from build123d import *

# Parameters (mm, degrees)
ESQUISSE1_W                  = 300
ESQUISSE1_H                  = 100
BOSS_EXTRU_1_DEPTH           = 1.5875
ESQUISSE2_W                  = 19.05
ESQUISSE2_H                  = 61.9
BOSS_EXTRU_2_DEPTH           = 1.5875
ESQUISSE3_W                  = 1.5875
ESQUISSE3_H                  = 61.9
BOSS_EXTRU_3_DEPTH           = 17.4625
ENL_V_MAT_EXTRU_1_REACH      = 5.175
ESQUISSE4_R                  = 1.5875
ENL_V_MAT_EXTRU_2_REACH      = 22.637
ESQUISSE5_R                  = 1.5875
ENL_V_MAT_EXTRU_3_REACH      = 22.637
ESQUISSE6_R                  = 1.5875
ESQUISSE7_R                  = 1.5875
ENL_V_MAT_EXTRU_4_DEPTH      = 297.825
ENL_V_MAT_EXTRU_4_DEPTH_BACK = 4.175


with BuildPart() as part:
    # Esquisse1 → Boss.-Extru.1 (new body)
    with BuildSketch(Plane.XY):
        with Locations((29.89832913, 31.147540984)):
            Rectangle(ESQUISSE1_W, ESQUISSE1_H)
    extrude(amount=BOSS_EXTRU_1_DEPTH)

    # Esquisse2 → Boss.-Extru.2 (add)
    with BuildSketch(Plane(origin=(0, 0, 0), x_dir=(-1, 0, 0), z_dir=(0, 0, -1))):
        with Locations((108.98917087, 31.147540984)):
            Rectangle(ESQUISSE2_W, ESQUISSE2_H)
        with Locations((-168.78582913, 31.147540984)):
            Rectangle(ESQUISSE2_W, ESQUISSE2_H)
    extrude(amount=BOSS_EXTRU_2_DEPTH)

    # Esquisse3 → Boss.-Extru.3 (add)
    with BuildSketch(Plane(origin=(0, 0, -1.5875), x_dir=(-1, 0, 0), z_dir=(0, 0, -1))):
        with Locations((-177.51707913, 31.147540984)):
            Rectangle(ESQUISSE3_W, ESQUISSE3_H)
        with Locations((117.72042087, 31.147540984)):
            Rectangle(ESQUISSE3_W, ESQUISSE3_H)
    extrude(amount=BOSS_EXTRU_3_DEPTH)

    # Esquisse4 → Enlèv. mat.-Extru.1 (cut, up to next)
    with BuildSketch(Plane(origin=(0, 0, -1.5875), x_dir=(-1, 0, 0), z_dir=(0, 0, -1)), mode=Mode.PRIVATE) as enl_v_mat_extru_1_sk1:
        with Locations((-167.99207913, 52.572540984)):
            Circle(ESQUISSE4_R)
    enl_v_mat_extru_1_tool1 = extrude(enl_v_mat_extru_1_sk1.sketch, amount=-ENL_V_MAT_EXTRU_1_REACH, mode=Mode.PRIVATE) & part.part
    add(enl_v_mat_extru_1_tool1.solids().sort_by_distance((167.992079, 52.572541, -1.5875))[0], mode=Mode.SUBTRACT)
    # Esquisse4 → Enlèv. mat.-Extru.1 (cut, up to next)
    with BuildSketch(Plane(origin=(0, 0, -1.5875), x_dir=(-1, 0, 0), z_dir=(0, 0, -1)), mode=Mode.PRIVATE) as enl_v_mat_extru_1_sk2:
        with Locations((-167.99207913, 9.722540984)):
            Circle(ESQUISSE4_R)
    enl_v_mat_extru_1_tool2 = extrude(enl_v_mat_extru_1_sk2.sketch, amount=-ENL_V_MAT_EXTRU_1_REACH, mode=Mode.PRIVATE) & part.part
    add(enl_v_mat_extru_1_tool2.solids().sort_by_distance((167.992079, 9.722541, -1.5875))[0], mode=Mode.SUBTRACT)
    # Esquisse4 → Enlèv. mat.-Extru.1 (cut, up to next)
    with BuildSketch(Plane(origin=(0, 0, -1.5875), x_dir=(-1, 0, 0), z_dir=(0, 0, -1)), mode=Mode.PRIVATE) as enl_v_mat_extru_1_sk3:
        with Locations((108.19542087, 52.572540984)):
            Circle(ESQUISSE4_R)
    enl_v_mat_extru_1_tool3 = extrude(enl_v_mat_extru_1_sk3.sketch, amount=-ENL_V_MAT_EXTRU_1_REACH, mode=Mode.PRIVATE) & part.part
    add(enl_v_mat_extru_1_tool3.solids().sort_by_distance((-108.195421, 52.572541, -1.5875))[0], mode=Mode.SUBTRACT)
    # Esquisse4 → Enlèv. mat.-Extru.1 (cut, up to next)
    with BuildSketch(Plane(origin=(0, 0, -1.5875), x_dir=(-1, 0, 0), z_dir=(0, 0, -1)), mode=Mode.PRIVATE) as enl_v_mat_extru_1_sk4:
        with Locations((108.19542087, 9.722540984)):
            Circle(ESQUISSE4_R)
    enl_v_mat_extru_1_tool4 = extrude(enl_v_mat_extru_1_sk4.sketch, amount=-ENL_V_MAT_EXTRU_1_REACH, mode=Mode.PRIVATE) & part.part
    add(enl_v_mat_extru_1_tool4.solids().sort_by_distance((-108.195421, 9.722541, -1.5875))[0], mode=Mode.SUBTRACT)

    # Esquisse5 → Enlèv. mat.-Extru.2 (cut, up to next)
    with BuildSketch(Plane.XY.offset(1.5875), mode=Mode.PRIVATE) as enl_v_mat_extru_2_sk1:
        with Locations((-108.19542087, -8.533709016)):
            Circle(ESQUISSE5_R)
    enl_v_mat_extru_2_tool1 = extrude(enl_v_mat_extru_2_sk1.sketch, amount=-ENL_V_MAT_EXTRU_2_REACH, mode=Mode.PRIVATE) & part.part
    add(enl_v_mat_extru_2_tool1.solids().sort_by_distance((-108.195421, -8.533709, 1.5875))[0], mode=Mode.SUBTRACT)
    # Esquisse5 → Enlèv. mat.-Extru.2 (cut, up to next)
    with BuildSketch(Plane.XY.offset(1.5875), mode=Mode.PRIVATE) as enl_v_mat_extru_2_sk2:
        with Locations((-89.93917087, -8.533709016)):
            Circle(ESQUISSE5_R)
    enl_v_mat_extru_2_tool2 = extrude(enl_v_mat_extru_2_sk2.sketch, amount=-ENL_V_MAT_EXTRU_2_REACH, mode=Mode.PRIVATE) & part.part
    add(enl_v_mat_extru_2_tool2.solids().sort_by_distance((-89.939171, -8.533709, 1.5875))[0], mode=Mode.SUBTRACT)
    # Esquisse5 → Enlèv. mat.-Extru.2 (cut, up to next)
    with BuildSketch(Plane.XY.offset(1.5875), mode=Mode.PRIVATE) as enl_v_mat_extru_2_sk3:
        with Locations((-30.02042087, -8.533709016)):
            Circle(ESQUISSE5_R)
    enl_v_mat_extru_2_tool3 = extrude(enl_v_mat_extru_2_sk3.sketch, amount=-ENL_V_MAT_EXTRU_2_REACH, mode=Mode.PRIVATE) & part.part
    add(enl_v_mat_extru_2_tool3.solids().sort_by_distance((-30.020421, -8.533709, 1.5875))[0], mode=Mode.SUBTRACT)
    # Esquisse5 → Enlèv. mat.-Extru.2 (cut, up to next)
    with BuildSketch(Plane.XY.offset(1.5875), mode=Mode.PRIVATE) as enl_v_mat_extru_2_sk4:
        with Locations((29.89832913, -8.533709016)):
            Circle(ESQUISSE5_R)
    enl_v_mat_extru_2_tool4 = extrude(enl_v_mat_extru_2_sk4.sketch, amount=-ENL_V_MAT_EXTRU_2_REACH, mode=Mode.PRIVATE) & part.part
    add(enl_v_mat_extru_2_tool4.solids().sort_by_distance((29.898329, -8.533709, 1.5875))[0], mode=Mode.SUBTRACT)
    # Esquisse5 → Enlèv. mat.-Extru.2 (cut, up to next)
    with BuildSketch(Plane.XY.offset(1.5875), mode=Mode.PRIVATE) as enl_v_mat_extru_2_sk5:
        with Locations((89.81707913, -8.533709016)):
            Circle(ESQUISSE5_R)
    enl_v_mat_extru_2_tool5 = extrude(enl_v_mat_extru_2_sk5.sketch, amount=-ENL_V_MAT_EXTRU_2_REACH, mode=Mode.PRIVATE) & part.part
    add(enl_v_mat_extru_2_tool5.solids().sort_by_distance((89.817079, -8.533709, 1.5875))[0], mode=Mode.SUBTRACT)
    # Esquisse5 → Enlèv. mat.-Extru.2 (cut, up to next)
    with BuildSketch(Plane.XY.offset(1.5875), mode=Mode.PRIVATE) as enl_v_mat_extru_2_sk6:
        with Locations((149.73582913, -8.533709016)):
            Circle(ESQUISSE5_R)
    enl_v_mat_extru_2_tool6 = extrude(enl_v_mat_extru_2_sk6.sketch, amount=-ENL_V_MAT_EXTRU_2_REACH, mode=Mode.PRIVATE) & part.part
    add(enl_v_mat_extru_2_tool6.solids().sort_by_distance((149.735829, -8.533709, 1.5875))[0], mode=Mode.SUBTRACT)
    # Esquisse5 → Enlèv. mat.-Extru.2 (cut, up to next)
    with BuildSketch(Plane.XY.offset(1.5875), mode=Mode.PRIVATE) as enl_v_mat_extru_2_sk7:
        with Locations((167.99207913, -8.533709016)):
            Circle(ESQUISSE5_R)
    enl_v_mat_extru_2_tool7 = extrude(enl_v_mat_extru_2_sk7.sketch, amount=-ENL_V_MAT_EXTRU_2_REACH, mode=Mode.PRIVATE) & part.part
    add(enl_v_mat_extru_2_tool7.solids().sort_by_distance((167.992079, -8.533709, 1.5875))[0], mode=Mode.SUBTRACT)
    # Esquisse5 → Enlèv. mat.-Extru.2 (cut, up to next)
    with BuildSketch(Plane.XY.offset(1.5875), mode=Mode.PRIVATE) as enl_v_mat_extru_2_sk8:
        with Locations((167.99207913, 70.828790984)):
            Circle(ESQUISSE5_R)
    enl_v_mat_extru_2_tool8 = extrude(enl_v_mat_extru_2_sk8.sketch, amount=-ENL_V_MAT_EXTRU_2_REACH, mode=Mode.PRIVATE) & part.part
    add(enl_v_mat_extru_2_tool8.solids().sort_by_distance((167.992079, 70.828791, 1.5875))[0], mode=Mode.SUBTRACT)
    # Esquisse5 → Enlèv. mat.-Extru.2 (cut, up to next)
    with BuildSketch(Plane.XY.offset(1.5875), mode=Mode.PRIVATE) as enl_v_mat_extru_2_sk9:
        with Locations((149.73582913, 70.828790984)):
            Circle(ESQUISSE5_R)
    enl_v_mat_extru_2_tool9 = extrude(enl_v_mat_extru_2_sk9.sketch, amount=-ENL_V_MAT_EXTRU_2_REACH, mode=Mode.PRIVATE) & part.part
    add(enl_v_mat_extru_2_tool9.solids().sort_by_distance((149.735829, 70.828791, 1.5875))[0], mode=Mode.SUBTRACT)
    # Esquisse5 → Enlèv. mat.-Extru.2 (cut, up to next)
    with BuildSketch(Plane.XY.offset(1.5875), mode=Mode.PRIVATE) as enl_v_mat_extru_2_sk10:
        with Locations((89.81707913, 70.828790984)):
            Circle(ESQUISSE5_R)
    enl_v_mat_extru_2_tool10 = extrude(enl_v_mat_extru_2_sk10.sketch, amount=-ENL_V_MAT_EXTRU_2_REACH, mode=Mode.PRIVATE) & part.part
    add(enl_v_mat_extru_2_tool10.solids().sort_by_distance((89.817079, 70.828791, 1.5875))[0], mode=Mode.SUBTRACT)
    # Esquisse5 → Enlèv. mat.-Extru.2 (cut, up to next)
    with BuildSketch(Plane.XY.offset(1.5875), mode=Mode.PRIVATE) as enl_v_mat_extru_2_sk11:
        with Locations((29.89832913, 70.828790984)):
            Circle(ESQUISSE5_R)
    enl_v_mat_extru_2_tool11 = extrude(enl_v_mat_extru_2_sk11.sketch, amount=-ENL_V_MAT_EXTRU_2_REACH, mode=Mode.PRIVATE) & part.part
    add(enl_v_mat_extru_2_tool11.solids().sort_by_distance((29.898329, 70.828791, 1.5875))[0], mode=Mode.SUBTRACT)
    # Esquisse5 → Enlèv. mat.-Extru.2 (cut, up to next)
    with BuildSketch(Plane.XY.offset(1.5875), mode=Mode.PRIVATE) as enl_v_mat_extru_2_sk12:
        with Locations((-30.02042087, 70.828790984)):
            Circle(ESQUISSE5_R)
    enl_v_mat_extru_2_tool12 = extrude(enl_v_mat_extru_2_sk12.sketch, amount=-ENL_V_MAT_EXTRU_2_REACH, mode=Mode.PRIVATE) & part.part
    add(enl_v_mat_extru_2_tool12.solids().sort_by_distance((-30.020421, 70.828791, 1.5875))[0], mode=Mode.SUBTRACT)
    # Esquisse5 → Enlèv. mat.-Extru.2 (cut, up to next)
    with BuildSketch(Plane.XY.offset(1.5875), mode=Mode.PRIVATE) as enl_v_mat_extru_2_sk13:
        with Locations((-89.93917087, 70.828790984)):
            Circle(ESQUISSE5_R)
    enl_v_mat_extru_2_tool13 = extrude(enl_v_mat_extru_2_sk13.sketch, amount=-ENL_V_MAT_EXTRU_2_REACH, mode=Mode.PRIVATE) & part.part
    add(enl_v_mat_extru_2_tool13.solids().sort_by_distance((-89.939171, 70.828791, 1.5875))[0], mode=Mode.SUBTRACT)
    # Esquisse5 → Enlèv. mat.-Extru.2 (cut, up to next)
    with BuildSketch(Plane.XY.offset(1.5875), mode=Mode.PRIVATE) as enl_v_mat_extru_2_sk14:
        with Locations((-108.19542087, 70.828790984)):
            Circle(ESQUISSE5_R)
    enl_v_mat_extru_2_tool14 = extrude(enl_v_mat_extru_2_sk14.sketch, amount=-ENL_V_MAT_EXTRU_2_REACH, mode=Mode.PRIVATE) & part.part
    add(enl_v_mat_extru_2_tool14.solids().sort_by_distance((-108.195421, 70.828791, 1.5875))[0], mode=Mode.SUBTRACT)

    # Esquisse6 → Enlèv. mat.-Extru.3 (cut, up to next)
    with BuildSketch(Plane.XY.offset(1.5875), mode=Mode.PRIVATE) as enl_v_mat_extru_3_sk1:
        with Locations((19.89832913, 31.147540984)):
            Circle(ESQUISSE6_R)
    enl_v_mat_extru_3_tool1 = extrude(enl_v_mat_extru_3_sk1.sketch, amount=-ENL_V_MAT_EXTRU_3_REACH, mode=Mode.PRIVATE) & part.part
    add(enl_v_mat_extru_3_tool1.solids().sort_by_distance((19.898329, 31.147541, 1.5875))[0], mode=Mode.SUBTRACT)

    # Esquisse7 → Enlèv. mat.-Extru.4 (cut, two sides)
    with BuildSketch(Plane.ZY.offset(-176.72332913)) as enl_v_mat_extru_4_sk:
        with Locations((-10.31875, 52.572540984)):
            Circle(ESQUISSE7_R)
        with Locations((-10.31875, 9.722540984)):
            Circle(ESQUISSE7_R)
    extrude(amount=ENL_V_MAT_EXTRU_4_DEPTH, mode=Mode.SUBTRACT)
    extrude(enl_v_mat_extru_4_sk.sketch, amount=-ENL_V_MAT_EXTRU_4_DEPTH_BACK, mode=Mode.SUBTRACT)


solid = part.part
For this review, take the finished solid that the model builds, in its own axes (mm). A direction names the side the tool comes from. Round coordinates to 2 decimals unless told otherwise and drop trailing zeros. Loops run counter-clockwise (first coordinate to the right, second up) from the corner with the lowest first, then second, coordinate; pieces in that order, holes last. Notation, with made-up numbers: (78.5, 21) - (85.5, 21) arc R5 ccw to (85.5, 28) - close; hole circle Ø11 at (-28, 76.25). An arc over 180 degrees is marked (long way). One line per item, written item: value. Start each with the question number.
Item 1: Take a section at B-B (z = -15.75). Give the boundary of the cut face in (x, y).
Item 2: The part is to be moulded in two halves that separate along X. For faces 5 (the flat face through (-113, 62.098, -1)), 6 (the flat face through (28, 32, 0)), 7 (the flat face through (178.311, 31, -9)), 8 (the flat face through (-118.514, 31, -9)), say which applies: +X half, -X half, draft (parallel to the pull), parting line (faces both ways), or undercut.
Item 3: For faces 1 (the flat face through (-116.927, 31, -10)), 2 (the flat face through (-113, 0.198, -1)), 3 (the flat face through (177, 62.098, -5)), 4 (the flat face through (28, 32, 1.588)), list the 3-axis set-ups (+Z, -Z, +X, -X, +Y, -Y) from which the entire face can be reached by the end or side of a thin tool; tool diameter is ignored.
Item 4: Clearance check with flat-ended pins moving along their axes: pin 1 Ø2.5 at (x, y) = (167.99, 52.57) entering from -Z; pin 2 Ø5 at (y, z) = (52.57, -10.32) entering from -X; pin 3 Ø3.5 at (y, z) = (9.72, -10.32) entering from +X; pin 4 Ø3.5 at (x, y) = (-89.94, 70.83) entering from -Z. State where each tip first meets the part, or that it passes through.
Item 5: Take a section at A-A (y = 19). Give the boundary of the cut face in (x, z), plus the area to 3 significant figures.
Item 6: For L1, parallel to X at y = 33, z = -4.5; L2, parallel to Z at x = 113, y = 37, list the stretches that pass through material, from the lowest coordinate up.
Item 7: Take a section at D-D (y = 75.5). Give the boundary of the cut face in (x, z), plus the area to 3 significant figures.
Item 8: Take a section at C-C (x = 131.5). Give the boundary of the cut face in (y, z), plus the area to 3 significant figures.
Answer below:
1. outline: (-118.51, 0.2) - (-116.93, 0.2) - (-116.93, 62.1) - (-118.51, 62.1) - close; (176.72, 0.2) - (178.31, 0.2) - (178.31, 62.1) - (176.72, 62.1) - close
2. face 5: draft
2. face 6: undercut
2. face 7: +X half
2. face 8: -X half
3. face 1: -Z, +Y, -Y
3. face 2: -Z, +X, -X, -Y
3. face 3: -Z, +X, -X, +Y
3. face 4: +Z, +X, -X, +Y, -Y
4. pin 1: passes through
4. pin 2: stops at x = -118.51
4. pin 3: stops at x = 178.31
4. pin 4: stops at z = 0
5. outline: (-120.1, 0) - (-118.51, 0) - (-118.51, -19.05) - (-116.93, -19.05) - (-116.93, -1.59) - (-99.46, -1.59) - (-99.46, 0) - (159.26, 0) - (159.26, -1.59) - (176.72, -1.59) - (176.72, -19.05) - (178.31, -19.05) - (178.31, 0) - (179.9, 0) - (179.9, 1.59) - (-120.1, 1.59) - close
5. area: 592 mm2
6. L1: x = -118.51 to -116.93, 176.72 to 178.31
6. L2: z = 0 to 1.59
7. outline: (-120.1, 0) - (179.9, 0) - (179.9, 1.59) - (-120.1, 1.59) - close
7. area: 476 mm2
8. outline: (-18.85, 0) - (81.15, 0) - (81.15, 1.59) - (-18.85, 1.59) - close
8. area: 159 mm2
